The figure shows three views and two pictorial views of one solid part (mm, origin at its lowest corner). Answer the questions. A direction names the side the tool comes from. Coordinates: 2 decimals unless noted, no trailing zeros. Write each loop counter-clockwise with the first axis right and the second up, starting at its lowest first coordinate (ties: lowest second). Pieces come first, ordered by that corner, then holes.
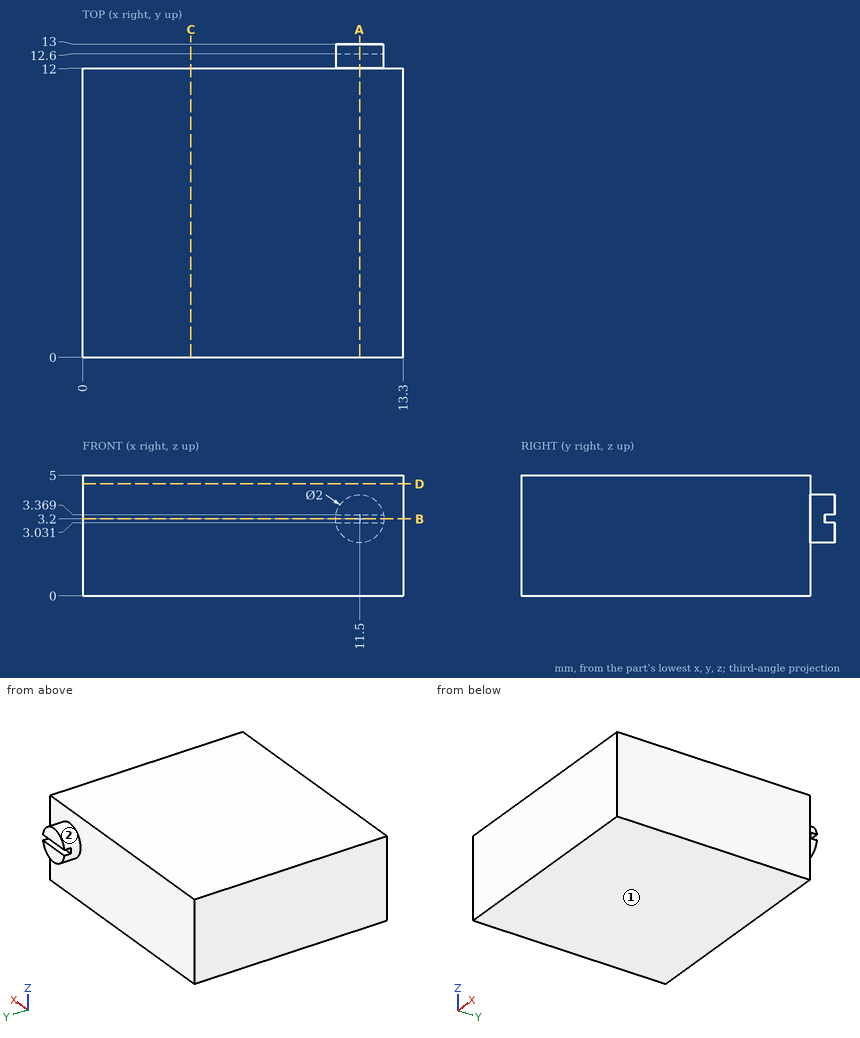
Q1. Find the intervals of material crossed by probe 1 along Y at (x, z) = (5, 2.25), in increasing order.
Answers below:
probe 1: y = 0 to 12
Q2. The part is cut by section C-C, the plane x = 4.5. Write down the section's boundary in (y, z).
Answers below:
outline: (0, 0) - (12, 0) - (12, 5) - (0, 5) - close
Q3. Which of the six approach directions +Z, -Z, +X, -X, +Y, -Y give full straight-line access (tool end or side, diameter ignored) to the marked faces 1 and 2?
Answers below:
face 1: -Z, +X, -X, +Y, -Y
face 2: +Y
Q4. The part is cut by section A-A, the plane x = 11.5. Write down the section's boundary in (y, z).
Answers below:
outline: (0, 0) - (12, 0) - (12, 2.2) - (13, 2.2) - (13, 3.03) - (12.6, 3.03) - (12.6, 3.37) - (13, 3.37) - (13, 4.2) - (12, 4.2) - (12, 5) - (0, 5) - close
Q5. The part is cut by section B-B, the plane z = 3.2. Write down the section's boundary in (x, y).
Answers below:
outline: (0, 0) - (13.3, 0) - (13.3, 12) - (12.5, 12) - (12.5, 12.6) - (10.5, 12.6) - (10.5, 12) - (0, 12) - close
Q6. The part is cut by section D-D, the plane z = 4.65. Write down the section's boundary in (x, y), then the cut area to 3 significant figures.
Answers below:
outline: (0, 0) - (13.3, 0) - (13.3, 12) - (0, 12) - close
area: 160 mm2
